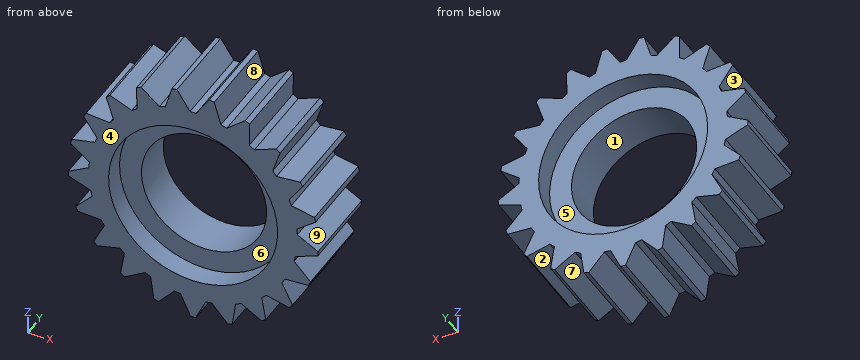
```python
from build123d import *

# Parameters (mm, degrees)
CUT_EXTRUDE1_DEPTH      = 47.904157598
CUT_EXTRUDE1_DEPTH_BACK = 47.904157598
SKETCH2_R               = 30


with BuildPart() as part:
    # Sketch1 → Revolve1 (revolve)
    with BuildSketch(Plane(origin=(0, 0, 0), x_dir=(0, 0, -1), z_dir=(1, 0, 0))):
        Polygon((20.25, 10), (30, 10), (30, -10), (20.25, -10), (20.25, -5), (15, -5), (15, 5), (20.25, 5), align=None)
    revolve(axis=Axis((0, 0, 0), (0, 1, 0)))

    # Sketch2 → Cut-Extrude1 (cut, two sides: drawn at the far end of the back side and taken through both)
    with BuildSketch(Plane(origin=(0, 10, 0), x_dir=(1, 0, 0), z_dir=(0, 1, 0)).offset(-CUT_EXTRUDE1_DEPTH_BACK)):
        Circle(SKETCH2_R)
        with BuildLine():
            Line((-3, 24.819347292), (-0.6, 29.978082123))
            Line((-0.6, 29.978082123), (0.6, 29.978082123))
            Line((0.6, 29.978082123), (3, 24.819347292))
            ThreePointArc((3, 24.819347292), (3.726056654, 24.720770656), (4.448912622, 24.600958853))
            Line((4.448912622, 24.600958853), (8.262851141, 28.823093151))
            Line((8.262851141, 28.823093151), (9.409538508, 28.469386942))
            Line((9.409538508, 28.469386942), (10.182349457, 22.832427806))
            ThreePointArc((10.182349457, 22.832427806), (10.847093478, 22.524221698), (11.502519835, 22.19666726))
            Line((11.502519835, 22.19666726), (16.391511698, 25.107045865))
            Line((16.391511698, 25.107045865), (17.382998227, 24.431061795))
            Line((17.382998227, 24.431061795), (16.459952481, 18.816746912))
            ThreePointArc((16.459952481, 18.816746912), (17.004318444, 18.326296796), (17.534077682, 17.820104373))
            Line((17.534077682, 17.820104373), (23.063714507, 19.160127373))
            Line((23.063714507, 19.160127373), (23.811902269, 18.221929594))
            Line((23.811902269, 18.221929594), (21.275016493, 13.129115478))
            ThreePointArc((21.275016493, 13.129115478), (21.650635095, 12.5), (22.007655779, 11.86014701))
            Line((22.007655779, 11.86014701), (27.686605069, 11.510747481))
            Line((27.686605069, 11.510747481), (28.125014298, 10.393698982))
            Line((28.125014298, 10.393698982), (24.199701926, 6.274904518))
            ThreePointArc((24.199701926, 6.274904518), (24.373197805, 5.563023349), (24.525757082, 4.846363537))
            Line((24.525757082, 4.846363537), (29.849419269, 2.838587161))
            Line((29.849419269, 2.838587161), (29.939095382, 1.641942604))
            Line((29.939095382, 1.641942604), (24.974137644, -1.136859246))
            ThreePointArc((24.974137644, -1.136859246), (24.93009493, -1.86825234), (24.864637239, -2.598040603))
            Line((24.864637239, -2.598040603), (29.359981576, -6.085794085))
            Line((29.359981576, -6.085794085), (29.092956455, -7.25570758))
            Line((29.092956455, -7.25570758), (23.529511635, -8.447608076))
            ThreePointArc((23.529511635, -8.447608076), (23.271843716, -9.133525609), (22.99418526, -9.811597435))
            Line((22.99418526, -9.811597435), (26.261780675, -14.469425819))
            Line((26.261780675, -14.469425819), (25.661780675, -15.508656304))
            Line((25.661780675, -15.508656304), (19.99418526, -15.007749857))
            ThreePointArc((19.99418526, -15.007749857), (19.545787062, -15.587245046), (19.080599013, -16.153350777))
            Line((19.080599013, -16.153350777), (20.830105314, -21.567385572))
            Line((20.830105314, -21.567385572), (19.950443068, -22.383592857))
            Line((19.950443068, -22.383592857), (14.682287782, -20.234387203))
            ThreePointArc((14.682287782, -20.234387203), (14.083001452, -20.655969358), (13.471617809, -21.059808014))
            Line((13.471617809, -21.059808014), (13.547583684, -26.748988469))
            Line((13.547583684, -26.748988469), (12.466421042, -27.269648956))
            Line((12.466421042, -27.269648956), (8.065804602, -23.663110449))
            ThreePointArc((8.065804602, -23.663110449), (7.36887936, -23.889320145), (6.665624244, -24.095008891))
            Line((6.665624244, -24.095008891), (5.061299791, -29.553826355))
            Line((5.061299791, -29.553826355), (3.8747028, -29.732677074))
            Line((3.8747028, -29.732677074), (0.732639287, -24.989262488))
            ThreePointArc((0.732639287, -24.989262488), (0, -25), (-0.732639287, -24.989262488))
            Line((-0.732639287, -24.989262488), (-3.8747028, -29.732677074))
            Line((-3.8747028, -29.732677074), (-5.061299791, -29.553826355))
            Line((-5.061299791, -29.553826355), (-6.665624244, -24.095008891))
            ThreePointArc((-6.665624244, -24.095008891), (-7.36887936, -23.889320145), (-8.065804602, -23.663110449))
            Line((-8.065804602, -23.663110449), (-12.466421042, -27.269648956))
            Line((-12.466421042, -27.269648956), (-13.547583684, -26.748988469))
            Line((-13.547583684, -26.748988469), (-13.471617809, -21.059808014))
            ThreePointArc((-13.471617809, -21.059808014), (-14.083001452, -20.655969358), (-14.682287782, -20.234387203))
            Line((-14.682287782, -20.234387203), (-19.950443068, -22.383592857))
            Line((-19.950443068, -22.383592857), (-20.830105314, -21.567385572))
            Line((-20.830105314, -21.567385572), (-19.080599013, -16.153350777))
            ThreePointArc((-19.080599013, -16.153350777), (-19.545787062, -15.587245046), (-19.99418526, -15.007749857))
            Line((-19.99418526, -15.007749857), (-25.661780675, -15.508656304))
            Line((-25.661780675, -15.508656304), (-26.261780675, -14.469425819))
            Line((-26.261780675, -14.469425819), (-22.99418526, -9.811597435))
            ThreePointArc((-22.99418526, -9.811597435), (-23.271843716, -9.133525609), (-23.529511635, -8.447608076))
            Line((-23.529511635, -8.447608076), (-29.092956455, -7.25570758))
            Line((-29.092956455, -7.25570758), (-29.359981576, -6.085794085))
            Line((-29.359981576, -6.085794085), (-24.864637239, -2.598040603))
            ThreePointArc((-24.864637239, -2.598040603), (-24.93009493, -1.86825234), (-24.974137644, -1.136859246))
            Line((-24.974137644, -1.136859246), (-29.939095382, 1.641942604))
            Line((-29.939095382, 1.641942604), (-29.849419269, 2.838587161))
            Line((-29.849419269, 2.838587161), (-24.525757082, 4.846363537))
            ThreePointArc((-24.525757082, 4.846363537), (-24.373197805, 5.563023349), (-24.199701926, 6.274904518))
            Line((-24.199701926, 6.274904518), (-28.125014298, 10.393698982))
            Line((-28.125014298, 10.393698982), (-27.686605069, 11.510747481))
            Line((-27.686605069, 11.510747481), (-22.007655779, 11.86014701))
            ThreePointArc((-22.007655779, 11.86014701), (-21.650635095, 12.5), (-21.275016493, 13.129115478))
            Line((-21.275016493, 13.129115478), (-23.811902269, 18.221929594))
            Line((-23.811902269, 18.221929594), (-23.063714507, 19.160127373))
            Line((-23.063714507, 19.160127373), (-17.534077682, 17.820104373))
            ThreePointArc((-17.534077682, 17.820104373), (-17.004318444, 18.326296796), (-16.459952481, 18.816746912))
            Line((-16.459952481, 18.816746912), (-17.382998227, 24.431061795))
            Line((-17.382998227, 24.431061795), (-16.391511698, 25.107045865))
            Line((-16.391511698, 25.107045865), (-11.502519835, 22.19666726))
            ThreePointArc((-11.502519835, 22.19666726), (-10.847093478, 22.524221698), (-10.182349457, 22.832427806))
            Line((-10.182349457, 22.832427806), (-9.409538508, 28.469386942))
            Line((-9.409538508, 28.469386942), (-8.262851141, 28.823093151))
            Line((-8.262851141, 28.823093151), (-4.448912622, 24.600958853))
            ThreePointArc((-4.448912622, 24.600958853), (-3.726056654, 24.720770656), (-3, 24.819347292))
        make_face(mode=Mode.SUBTRACT)
    extrude(amount=CUT_EXTRUDE1_DEPTH + CUT_EXTRUDE1_DEPTH_BACK, mode=Mode.SUBTRACT)


solid = part.part
```
Here's how the part is built. I have some questions about the finished solid (model axes, mm). Face numbers are marked on the shaded views. A direction names the side the tool comes from. Give positions to 0.01 mm unless a question says otherwise; leave off trailing zeros. Order: outer loops, then holes, each group sorted by start corner. A loop starts at its lowest first (then second) coordinate and runs counter-clockwise, first axis right, second up. Notation, with made-up numbers: (-17.75, -2.5) - (27.25, -2.5) arc R21 ccw to (27.25, 15.5) - close; hole circle Ø11 at (-2, 67). An arc over 180 degrees is marked (long way). Answer as a JSON object with one key per item and string values. Group by question number.
Item 1: Please list where these lines run through material, in increasing order: probe 1 along Z at (x, y) = (0, -4.25); probe 2 along Z at (x, y) = (0, 8.9); probe 3 along X at (y, z) = (-5, -23.5).
Item 2: If we section it at A-A on z = 0: Please give me the cut outline in (x, y).
Item 3: If we mould it in two halves opening along Z, with no side actions, what happens to the marked faces 1, 2, 3 and 4? For each: pulls with the +Z half, pulls with the -Z half, needs draft (parallel to the pull), parting line crosses it, or undercut.
Item 4: For P1, Ø12, axis at x = -5, z = 8, coming from the -Y side; P2, Ø24, axis at x = 0, z = 0, coming from the +Y side; P3, Ø12, axis at x = -20, y = 1.5, coming from the -Z side; P4, Ø6, axis at x = 23, y = 6.5, coming from the +Z side, each with a flat end and sliding along its axis, tell me the tip position at first contact or that it passes through.
Item 5: Which directions (+Z, -Z, +X, -X, +Y, -Y) give clear straight access to the entire face, cutting with the end or side of a thin tool? Please do the marked faces 5, 6, 7, 8 and 9.
Result set:
{
 "1": {"probe 1": "-29.98 to -15, 15 to 25", "probe 2": "-29.98 to -20.25, 20.25 to 25", "probe 3": "-17.23 to -13.69, -10.09 to 10.09, 13.69 to 17.23"},
 "2": {"outline": "(-27.01, -10) - (-20.25, -10) - (-20.25, -5) - (-15, -5) - (-15, 5) - (-20.25, 5) - (-20.25, 10) - (-27.01, 10) - close; (15, -5) - (20.25, -5) - (20.25, -10) - (27.01, -10) - (27.01, 10) - (20.25, 10) - (20.25, 5) - (15, 5) - close"},
 "3": {"face 1": "undercut", "face 2": "pulls with the -Z half", "face 3": "undercut", "face 4": "needs draft"},
 "4": {"P1": "y = -5", "P2": "through", "P3": "z = -25.11", "P4": "z = 22.34"},
 "5": {"face 5": "+Y", "face 6": "-Y", "face 7": "-Z, +Y, -Y", "face 8": "+Z, +Y, -Y", "face 9": "+X, +Y, -Y"}
}
